from build123d import *


with BuildPart() as part:
    # Sketch1 → Revolve1 (revolve)
    with BuildSketch(Plane.XY):
        Polygon((0, 0), (-255.905, 0), (-255.905, 14.605), (-247.523, 14.605), (-242.758863359, 32.385), (-27.207318539, 32.385), (-26.52672759, 34.925), (-13.82672759, 34.925), (-8.382, 14.605), (0, 14.605), align=None)
    revolve(axis=Axis((0, 0, 0), (-1, 0, 0)))


solid = part.part
Design review of the part built by this model. Coordinates are the model's own, in mm. A direction names the side the tool comes from. Coordinates: 2 decimals unless noted, no trailing zeros. Order: outer loops, then holes, each group sorted by start corner. A loop starts at its lowest first (then second) coordinate and runs counter-clockwise, first axis right, second up. Notation, with made-up numbers: (42.5, 56) - (78.5, 56) arc R13 cw to (78.5, 63) - close; hole circle Ø2 at (72, -24.5). An arc over 180 degrees is marked (long way). Put each result on its own line as item: value.
1) Insertion check: P1, Ø4, axis at x = -60.5, z = 26, coming from the +Y side; P2, Ø4, axis at x = -181, z = 15, coming from the -Y side; P3, Ø10, axis at x = -45.5, y = -3, coming from the +Z side (3 decimals). Each pin has a flat end and moves straight along its axis. Give the tip position at first contact, or say it passes through.
Response values:
P1: stops at y = 21.74
P2: stops at y = -29.66
P3: stops at z = 32.385
2) Take a section at A-A, the plane y = 0. Give the boundary of the cut face in (x, z) (3 decimals), and give its area (3 significant figures).
Response values:
outline: (-255.905, -14.605) - (-247.523, -14.605) - (-242.759, -32.385) - (-27.207, -32.385) - (-26.527, -34.925) - (-13.827, -34.925) - (-8.382, -14.605) - (0, -14.605) - (0, 14.605) - (-8.382, 14.605) - (-13.827, 34.925) - (-26.527, 34.925) - (-27.207, 32.385) - (-242.759, 32.385) - (-247.523, 14.605) - (-255.905, 14.605) - close
area: 15,900 mm²
3) Take a section at C-C, the plane x = -106.5. Give the boundary of the cut face in (y, z) (3 decimals), and give its area (3 significant figures).
Response values:
outline: circle Ø64.77 at (0, 0)
area: 3,290 mm²
4) Wall thickness on L1, parallel to Z at x = -192, y = 1.5; L2, parallel to Y at x = -70, z = 0.5; L3, parallel to Z at x = -214, y = -1: over which ranges is each line inside the solid? List them lowest first. Write a range as from..to.
Response values:
L1: z = -32.35..32.35
L2: y = -32.38..32.38
L3: z = -32.37..32.37
5) Tool access review of faces 1 (the face through (-20.088, -27.715, 21.251)), 2 (the face through (-4.132, -10.764, -9.871)), 3 (the face through (-251.655, -10.764, -9.871)): name each direction out of +Z, -Z, +X, -X, +Y, -Y from which nothing blocks a thin tool from reaching the whole face with its end or side.
Response values:
face 1: +X, -X
face 2: +X
face 3: -X
